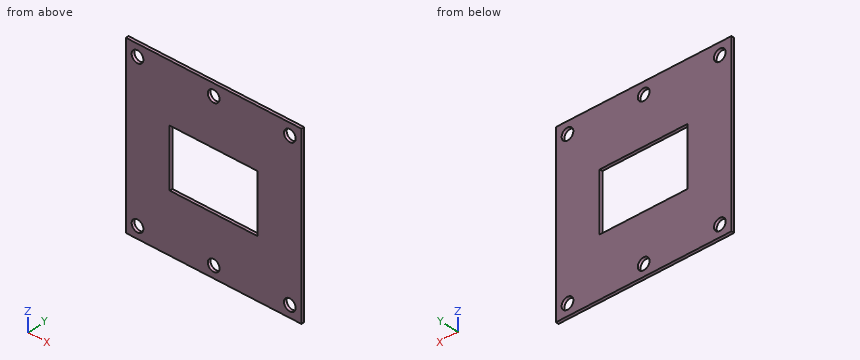
```python
from build123d import *

# Parameters (mm, degrees)
SKETCH1_W                    = 60
SKETCH1_H                    = 60
BOSS_EXTRUDE1_DEPTH          = 1
F_4_0_4_DIAMETER_HOLE1_D     = 4
F_4_0_4_DIAMETER_HOLE1_DEPTH = 1
SKETCH14_W                   = 30
SKETCH14_H                   = 20
CUT_EXTRUDE1_DEPTH           = 10


with BuildPart() as part:
    # Sketch1 → Boss-Extrude1 (new body)
    with BuildSketch(Plane(origin=(0, 0, 0), x_dir=(1, 0, 0), z_dir=(0, 1, 0))):
        Rectangle(SKETCH1_W, SKETCH1_H)
    extrude(amount=BOSS_EXTRUDE1_DEPTH)

    # Ø4.0 (4) Diameter Hole1
    with Locations(Plane(origin=(0, 1, 0), x_dir=(1, 0, 0), z_dir=(0, 1, 0))):
        with Locations((26, 26), (0, 26), (-26, 26), (0, -26), (26, -26), (-26, -26)):
            Hole(F_4_0_4_DIAMETER_HOLE1_D / 2, depth=F_4_0_4_DIAMETER_HOLE1_DEPTH)

    # Sketch14 → Cut-Extrude1 (cut)
    with BuildSketch(Plane(origin=(0, 1, 0), x_dir=(1, 0, 0), z_dir=(0, 1, 0))):
        Rectangle(SKETCH14_W, SKETCH14_H)
    extrude(amount=-CUT_EXTRUDE1_DEPTH, mode=Mode.SUBTRACT)


solid = part.part
```
Model file for the job. Use its own axes, mm. Give positions to 0.01 mm unless a question says otherwise; leave off trailing zeros. Write each loop counter-clockwise with the first axis right and the second up, starting at its lowest first coordinate (ties: lowest second). Pieces come first, ordered by that corner, then holes. Notation, with made-up numbers: (27.5, 24) -> (42.5, 24) arc R23 cw to (42.5, 63) -> close; hole circle Ø4 at (23, 13.25). An arc over 180 degrees is marked (long way). Use CSV: the item, a comma, the result in double quotes. Start each with the question number.
1) Cut at A-A on z = 4.5. List the corners of the cut face in (x, y).
2) Drill centre lines: L1, parallel to X at y = 0.4, z = -26; L2, parallel to Z at x = 26, y = 0.2; L3, parallel to Z at x = -12.5, y = 0.1. Where is each one in solid material? Low to high.
3) Cut at D-D on x = -26. List the corners of the cut face in (y, z), plus the area to 3 significant figures.
4) Cut at C-C on z = 26. List the corners of the cut face in (x, y).
5) Cut at B-B on x = 0. List the corners of the cut face in (y, z).
Final values:
1,outline,"(-30, 0) -> (-15, 0) -> (-15, 1) -> (-30, 1) -> close; (15, 0) -> (30, 0) -> (30, 1) -> (15, 1) -> close"
2,L1,"x = -30 to -28, -24 to -2, 2 to 24, 28 to 30"
2,L2,"z = -30 to -28, -24 to 24, 28 to 30"
2,L3,"z = -30 to -10, 10 to 30"
3,outline,"(0, -30) -> (1, -30) -> (1, -28) -> (0, -28) -> close; (0, -24) -> (1, -24) -> (1, 24) -> (0, 24) -> close; (0, 28) -> (1, 28) -> (1, 30) -> (0, 30) -> close"
3,area,"52.0 mm2"
4,outline,"(-30, 0) -> (-28, 0) -> (-28, 1) -> (-30, 1) -> close; (-24, 0) -> (-2, 0) -> (-2, 1) -> (-24, 1) -> close; (2, 0) -> (24, 0) -> (24, 1) -> (2, 1) -> close; (28, 0) -> (30, 0) -> (30, 1) -> (28, 1) -> close"
5,outline,"(0, -30) -> (1, -30) -> (1, -28) -> (0, -28) -> close; (0, -24) -> (1, -24) -> (1, -10) -> (0, -10) -> close; (0, 10) -> (1, 10) -> (1, 24) -> (0, 24) -> close; (0, 28) -> (1, 28) -> (1, 30) -> (0, 30) -> close"
